from build123d import *

# Parameters (mm, degrees)
SKETCH1_R           = 19
BOSS_EXTRUDE1_DEPTH = 3
SKETCH2_R           = 2
CUT_EXTRUDE1_DEPTH  = 3
SKETCH3_R           = 9
CUT_EXTRUDE2_DEPTH  = 3


with BuildPart() as part:
    # Sketch1 → Boss-Extrude1 (new body)
    with BuildSketch(Plane(origin=(0, 0, 0), x_dir=(1, 0, 0), z_dir=(0, 1, 0))):
        Circle(SKETCH1_R)
    extrude(amount=BOSS_EXTRUDE1_DEPTH)

    # Sketch2 → Cut-Extrude1 (cut)
    with BuildSketch(Plane(origin=(0, 3, 0), x_dir=(1, 0, 0), z_dir=(0, 1, 0))):
        with Locations((-11.974482975, 10.611868708)):
            Circle(SKETCH2_R)
        with Locations((10.611868708, 11.974482975)):
            Circle(SKETCH2_R)
        with Locations((11.974482975, -10.611868708)):
            Circle(SKETCH2_R)
        with Locations((-10.611868708, -11.974482975)):
            Circle(SKETCH2_R)
    extrude(amount=-CUT_EXTRUDE1_DEPTH, mode=Mode.SUBTRACT)

    # Sketch3 → Cut-Extrude2 (cut)
    with BuildSketch(Plane(origin=(0, 3, 0), x_dir=(1, 0, 0), z_dir=(0, 1, 0))):
        Circle(SKETCH3_R)
    extrude(amount=-CUT_EXTRUDE2_DEPTH, mode=Mode.SUBTRACT)


solid = part.part
Input: part model. Units: mm. Frame: model coordinates. Round coordinates to 2 decimals unless told otherwise and drop trailing zeros. Write each loop counter-clockwise with the first axis right and the second up, starting at its lowest first coordinate (ties: lowest second). Pieces come first, ordered by that corner, then holes.
1) Contact query for flat-ended pins moving along their axis: P1, Ø3, axis at x = 10.61, z = -11.97, coming from the +Y side; P2, Ø1.5, axis at y = 1, z = 7, coming from the -X side; P3, Ø1, axis at y = 1.5, z = 1.5, coming from the -X side. Output: stop coordinate, or through.
2) Cut plane D-D (z = 15). Return the cut outline in (x, y).
3) Cut plane B-B (x = 0). Return the cut outline in (y, z), then the cut area to 3 significant figures.
4) Draft query along Z for faces 1 (the cylindrical face through (8.767, 1.479, 16.856)), 2 (the flat face through (8.2, 0, -4.5)), 3 (the cylindrical face through (-12.086, 1.521, 10.623)). Return one class per face: pulls with the +Z half, pulls with the -Z half, needs draft (parallel to the pull), parting line crosses it, or undercut.
5) Cut plane C-C (y = 1.2). Return the cut outline in (x, z).
6) Cut plane A-A (z = 0). Return the cut outline in (x, y).
7) Ray query, L1, parallel to Z at x = 0, y = 2.25; L2, parallel to X at y = 1.15, z = 10.5. Return the intervals inside material, ascending.
Geometry says:
1. P1: passes through
1. P2: stops at x = -17.94
1. P3: stops at x = -18.97
2. outline: (-11.66, 0) - (11.66, 0) - (11.66, 3) - (-11.66, 3) - close
3. outline: (0, -19) - (3, -19) - (3, -9) - (0, -9) - close; (0, 9) - (3, 9) - (3, 19) - (0, 19) - close
3. area: 60.0 mm2
4. face 1: parting line crosses it
4. face 2: needs draft
4. face 3: undercut
5. outline: circle Ø38 at (0, 0); hole circle Ø4 at (-11.97, -10.61); hole circle Ø4 at (-10.61, 11.97); hole circle Ø18 at (0, 0); hole circle Ø4 at (10.61, -11.97); hole circle Ø4 at (11.97, 10.61)
6. outline: (-19, 0) - (-9, 0) - (-9, 3) - (-19, 3) - close; (9, 0) - (19, 0) - (19, 3) - (9, 3) - close
7. L1: z = -19 to -9, 9 to 19
7. L2: x = -15.84 to -11.96, -9.26 to 9.98, 13.97 to 15.84
